Design review of the part built by this model. Coordinates are the model's own, in mm. A direction names the side the tool comes from. Coordinates: 2 decimals unless noted, no trailing zeros. Loops run counter-clockwise (first coordinate to the right, second up) from the corner with the lowest first, then second, coordinate; pieces in that order, holes last.
Q1. Wall thickness on probe 1 along X at (y, z) = (19, 77.5); probe 2 along Z at (x, y) = (22.5, 56); probe 3 along Z at (x, y) = (45, 10.5): over which ranges is each line inside the solid? List them lowest first.
Q2. Machinability: for faces 1 (the face through (13.539, 8.543, 82.782)), 2 (the face through (25, 30, 30)), 3 (the face through (86, 50, 9)), 4 (the face through (14, 50, 83)), 5 (the face through (50, 25, 101)), which of the approach directions +Z, -Z, +X, -X, +Y, -Y give a long, thin tool a straight path to every point of the face, cutting with its end or side? Answer none if there is none.
Q3. Add section A-A on z = 124. Give the boundary of the cut face in (x, y), and give its area (3 significant figures).
Q4. Draft analysis for pull direction X (two halves, no side actions). For faces 6 (the face through (35.761, 8.543, 117.218)), 7 (the face through (25, 15, 60)), 8 (the face through (14.239, 44.584, 117.218)), state which applies: released by +X, released by -X, zero draft, split by the parting line, or undercut.
Q5. Add section D-D on z = 68.5. Give the boundary of the cut face in (x, y) (1 decimal), and give its area (3 significant figures).
Q6. Add section B-B on x = 87. Give the boundary of the cut face in (y, z), and give its area (3 significant figures).
Q7. For P1, Ø25, axis at y = 23, z = 103.5, coming from the +X side; P2, Ø4, axis at x = 26.5, z = 124.5, coming from the -Y side; P3, Ø2, axis at x = 13.5, y = 19, coming from the -Z side, all flat-tipped, find the tip position at first contact; note any pin that passes through.
```python
from build123d import *

# Parameters (mm, degrees)
F0_W      = 100
F0_H      = 100
F1_DEPTH  = 140
F3_DEPTH  = 140.001
F5_DEPTH  = 80
F9_DEPTH  = 50.00099999
F11_DEPTH = 50.00099999
F6_W      = 50
F6_H      = 80
F14_W     = 30
F14_H     = 60
F16_DEPTH = 49.99


with BuildPart() as f1:
    # F0 (on Top) → F1 (new body)
    with BuildSketch(Plane.XY):
        with Locations((50, 50)):
            Rectangle(F0_W, F0_H)
    extrude(amount=F1_DEPTH)

    # F2 (on face) → F3 (cut, through all)
    with BuildSketch(Plane.XY.offset(140)):
        with BuildLine():
            ThreePointArc((0, 50), (14.6446609407, 85.3553390593), (50, 100))
            Line((50, 100), (0, 100))
            Line((0, 100), (0, 50))
        make_face()
        with BuildLine():
            ThreePointArc((50, 100), (85.3553390593, 85.3553390593), (100, 50))
            Line((100, 50), (100, 100))
            Line((100, 100), (50, 100))
        make_face()
        with BuildLine():
            Line((100, 0), (100, 50))
            ThreePointArc((100, 50), (85.3553390593, 14.6446609407), (50, 0))
            Line((50, 0), (100, 0))
        make_face()
    extrude(amount=-F3_DEPTH, mode=Mode.SUBTRACT)

    # F4 (on face) → F5 (cut)
    with BuildSketch(Plane.XY.offset(140)):
        with BuildLine():
            ThreePointArc((100, 50), (50, 100), (0, 50))
            Line((0, 50), (50, 50))
            Line((50, 50), (50, 0))
            ThreePointArc((50, 0), (85.3553390593, 14.6446609407), (100, 50))
        make_face()
    extrude(amount=-F5_DEPTH, mode=Mode.SUBTRACT)

    # F8 (on face) → F9 (cut, through all)
    with BuildSketch(Plane.XZ.offset(-50)):
        Polygon((100, 60), (50.001, 60), (100, 30), align=None)
    extrude(amount=F9_DEPTH, mode=Mode.SUBTRACT)

    # F10 (on face) → F11 (cut, through all)
    with BuildSketch(Plane.XZ.offset(-50)):
        Polygon((50.001, 0), (100, 0), (100, 29.99), align=None)
    extrude(amount=-F11_DEPTH, mode=Mode.SUBTRACT)

    # F6 (on face) → F13 section 0
    with BuildSketch(Plane.XZ, mode=Mode.PRIVATE) as f13_s0:
        with Locations((25, 100)):
            Rectangle(F6_W, F6_H)
    loft([f13_s0.sketch, Vertex(0, 30, 140)], mode=Mode.SUBTRACT)

    # F14 (on face) → F16 (cut)
    with BuildSketch(Plane(origin=(0, 0, 0), x_dir=(0, -1, 0), z_dir=(-1, 0, 0))):
        with Locations((-15, 30)):
            Rectangle(F14_W, F14_H)
    extrude(amount=-F16_DEPTH, mode=Mode.SUBTRACT)

    # F17 (on face) → F18 section 0
    with BuildSketch(Plane.XY.offset(140), mode=Mode.PRIVATE) as f18_s0:
        Polygon((0, 50), (0, 30), (50, 50), align=None)
    loft([f18_s0.sketch, Vertex(50, 50, 60)], mode=Mode.SUBTRACT)


solid = f1.part
```
Entries:
1. probe 1: x = 0 to 50
1. probe 2: z = 0 to 60
1. probe 3: z = 60 to 140
2. face 1: +Z, -X, -Y
2. face 2: -Z, -X, -Y
2. face 3: -Z, +X, +Y
2. face 4: +Z, +X, -X, +Y
2. face 5: +Z, +X, +Y, -Y
3. outline: (0, 24) - (10, 24) - (50, 0) - (50, 50) - (10, 34) - (10, 50) - (0, 50) - close
3. area: 1,460 mm2
4. face 6: released by -X
4. face 7: zero draft
4. face 8: undercut
5. outline: (0, 3.2) - (44.7, 3.2) - (50, 0) - (50, 50) - (44.7, 47.9) - (44.7, 50) - (0, 50) - close
5. area: 2,340 mm2
6. outline: (16.37, 0) - (50, 0) - (50, 22.19) - (83.63, 22.19) - (83.63, 60) - (50, 60) - (50, 37.8) - (16.37, 37.8) - close
6. area: 2,540 mm2
7. P1: stops at x = 50
7. P2: stops at y = 12.9
7. P3: stops at z = 60
